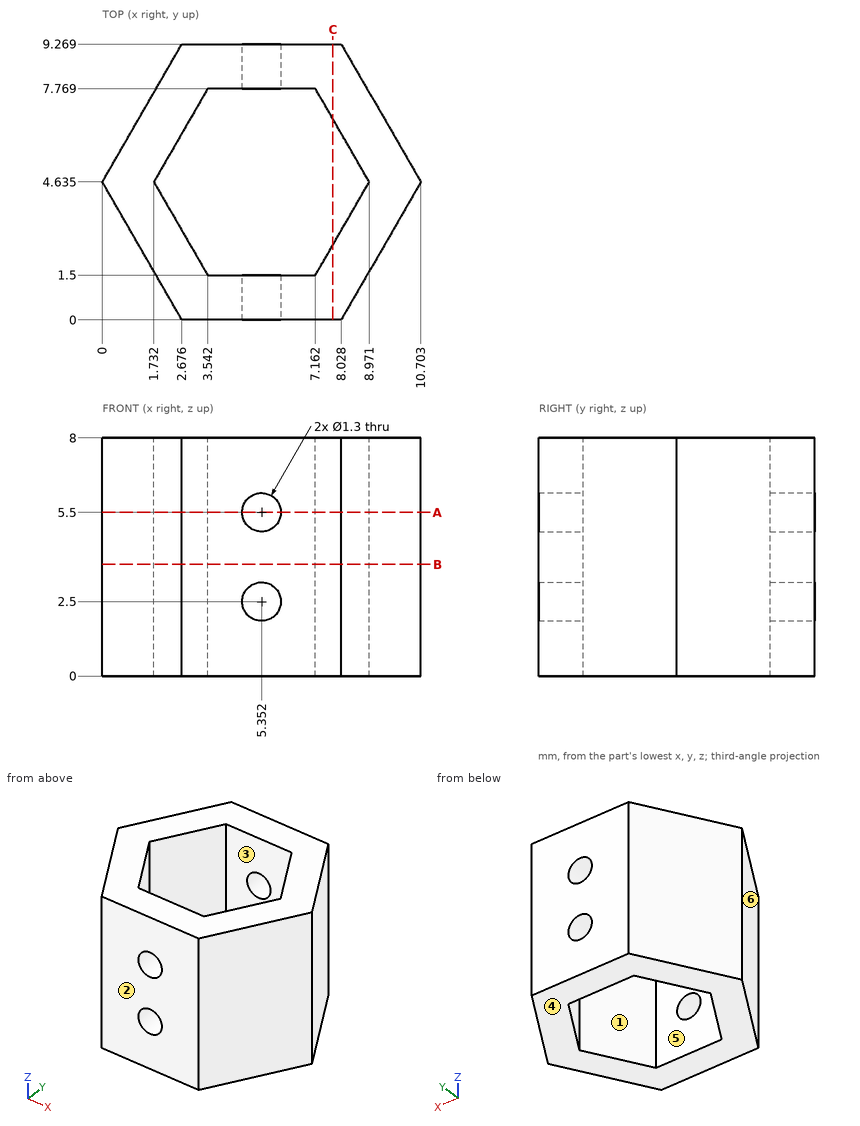
For this review, use the dimensioned drawing (mm, ordinates from the lowest corner) and the shaded views. A direction names the side the tool comes from. Coordinates: 2 decimals unless noted, no trailing zeros. Write each loop counter-clockwise with the first axis right and the second up, starting at its lowest first coordinate (ties: lowest second). Pieces come first, ordered by that corner, then holes. Notation, with made-up numbers: (33.5, 28.5) - (42.5, 28.5) arc R14 cw to (42.5, 44.5) - close; hole circle Ø7 at (28.25, 25). An arc over 180 degrees is marked (long way). Answer in a Markdown table with one row per item. Add a question column.
Q1. Clearance check with flat-ended pins moving along their axes: pin 1 (2 mm diameter, centred on y = 2, z = 4, fed in from +X); pin 2 (2 mm diameter, centred on x = 5.35, z = 5.5, fed in from +Y); pin 3 (1 mm diameter, centred on x = 3, y = 4.5, fed in from -Z); pin 4 (2 mm diameter, centred on x = 1.5, z = 5.5, fed in from -Y) (1 decimal). State where each tip first meets the part, or that it passes through.
Q2. Consider section C-C on x = 7.75. Give the boundary of the cut face in (y, z).
Q3. Draft analysis for pull direction Y (two halves, no side actions). For the marked faces 3, 4, 5 and 6, state which applies: +Y half, -Y half, draft (parallel to the pull), parting line (faces both ways), or undercut.
Q4. To check wall thickness, follow line 1 along Y through (x, z) = (7, 2); line 2 along X through (y, z) = (8.5, 6) (1 decimal); line 3 along Y through (x, z) = (2.5, 5.5) (1 decimal). State the ranges of each line that lie inside material, in increasing order. Write a range as from..to.
Q5. Consider section A-A on z = 5.5. Give the boundary of the cut face in (x, y) (1 decimal).
Q6. Consider section B-B on z = 3.75. Give the boundary of the cut face in (x, y) (1 decimal).
Q7. For the marked faces 1 and 2, list the 3-axis set-ups (+Z, -Z, +X, -X, +Y, -Y) from which the entire face can be reached by the end or side of a thin tool; tool diameter is ignored.
Answers below:
| question | item | result |
|---|---|---|
| 1 | pin 1 | x = 9.76 |
| 1 | pin 2 | y = 9.27 |
| 1 | pin 3 | through |
| 1 | pin 4 | y = 0.3 |
| 2 | outline | (0, 0) - (2.52, 0) - (2.52, 8) - (0, 8) - close; (6.75, 0) - (9.27, 0) - (9.27, 8) - (6.75, 8) - close |
| 3 | face 3 | undercut |
| 3 | face 4 | draft |
| 3 | face 5 | undercut |
| 3 | face 6 | -Y half |
| 4 | line 1 | 0..1.5, 7.77..9.27 |
| 4 | line 2 | 2.2..4.9, 5.8..8.5 |
| 4 | line 3 | 0.3..3.3, 6..9 |
| 5 | outline | (0, 4.6) - (2.7, 0) - (4.7, 0) - (4.7, 1.5) - (3.5, 1.5) - (1.7, 4.6) - (3.5, 7.8) - (4.7, 7.8) - (4.7, 9.3) - (2.7, 9.3) - close; (6, 0) - (8, 0) - (10.7, 4.6) - (8, 9.3) - (6, 9.3) - (6, 7.8) - (7.2, 7.8) - (9, 4.6) - (7.2, 1.5) - (6, 1.5) - close |
| 6 | outline | (0, 4.6) - (2.7, 0) - (8, 0) - (10.7, 4.6) - (8, 9.3) - (2.7, 9.3) - close; hole (1.7, 4.6) - (3.5, 1.5) - (7.2, 1.5) - (9, 4.6) - (7.2, 7.8) - (3.5, 7.8) - close |
| 7 | face 1 | +Z, -Z |
| 7 | face 2 | +Z, -Z, +X, -X, -Y |
